Geometry: final body of the model. Coordinates: model frame, mm. Face numbers are marked on the shaded views. Round coordinates to 2 decimals unless told otherwise and drop trailing zeros. Loops run counter-clockwise (first coordinate to the right, second up) from the corner with the lowest first, then second, coordinate; pieces in that order, holes last. Notation, with made-up numbers: (1, -15.5) - (54, -15.5) arc R20 cw to (54, 15.5) - close; hole circle Ø11 at (-19, -31.75). An arc over 180 degrees is marked (long way). Answer as CSV lines item,"result".
from build123d import *

# Parameters (mm, degrees)
BOSS_EXTRUDE1_DEPTH = 2.5
SKETCH3_R           = 2.25
SKETCH3_R_2         = 2.1
SKETCH3_R_3         = 2.121320344
CUT_EXTRUDE1_DEPTH  = 3
SKETCH4_R           = 33.5
SKETCH4_R_2         = 2.25
CUT_EXTRUDE2_DEPTH  = 5
CUT_EXTRUDE3_DEPTH  = 1.5
CHAMFER1_SIZE       = 2
CUT_EXTRUDE4_DEPTH  = 3
SKETCH7_R           = 2.25
SKETCH7_R_2         = 1.25
BOSS_EXTRUDE2_DEPTH = 3
CHAMFER2_SIZE       = 2
SKETCH12_W          = 9
SKETCH12_H          = 42.1
CUT_EXTRUDE5_DEPTH  = 7
CHAMFER3_SIZE       = 0.4


with BuildPart() as part:
    # Sketch1 → Boss-Extrude1 (new body)
    with BuildSketch(Plane.XY):
        with BuildLine():
            Line((-15.633211847, 85.984955899), (119.366788153, 85.984955899))
            ThreePointArc((119.366788153, 85.984955899), (126.437855965, 83.05602371), (129.366788153, 75.984955899))
            Line((129.366788153, 75.984955899), (129.366788153, 10.984955899))
            ThreePointArc((129.366788153, 10.984955899), (126.437855965, 3.913888087), (119.366788153, 0.984955899))
            Line((119.366788153, 0.984955899), (-15.633211847, 0.984955899))
            ThreePointArc((-15.633211847, 0.984955899), (-22.704279659, 3.913888087), (-25.633211847, 10.984955899))
            Line((-25.633211847, 10.984955899), (-25.633211847, 75.984955899))
            ThreePointArc((-25.633211847, 75.984955899), (-22.704279659, 83.05602371), (-15.633211847, 85.984955899))
        make_face()
    extrude(amount=BOSS_EXTRUDE1_DEPTH)

    # Sketch3 → Cut-Extrude1 (cut)
    with BuildSketch(Plane.XY.offset(2.5)):
        with Locations((119.266788153, 11.084955899)):
            Circle(SKETCH3_R)
        with Locations((119.266788153, 75.984955899)):
            Circle(SKETCH3_R_2)
        with Locations((-15.533211847, 75.984955899)):
            Circle(SKETCH3_R_3)
        with Locations((-15.533211847, 11.084955899)):
            Circle(SKETCH3_R_2)
    extrude(amount=-CUT_EXTRUDE1_DEPTH, mode=Mode.SUBTRACT)

    # Sketch4 → Cut-Extrude2 (cut)
    with BuildSketch(Plane.XY.offset(2.5)):
        with Locations((58.842502754, 40.410046739)):
            Circle(SKETCH4_R)
        with Locations((28.842502754, 70.410046739)):
            Circle(SKETCH4_R_2)
        with Locations((88.842502754, 70.410046739)):
            Circle(SKETCH4_R_2)
        with Locations((88.842502754, 10.410046739)):
            Circle(SKETCH4_R_2)
        with Locations((28.842502754, 10.410046739)):
            Circle(SKETCH4_R_2)
    extrude(amount=-CUT_EXTRUDE2_DEPTH, mode=Mode.SUBTRACT)

    # Sketch5 → Cut-Extrude3 (cut)
    with BuildSketch(Plane(origin=(0, 0, 0), x_dir=(-1, 0, 0), z_dir=(0, 0, -1))):
        Polygon((-93.172629773, 10.410046739), (-91.007566263, 6.660046739), (-86.677439244, 6.660046739), (-84.512375735, 10.410046739), (-86.677439244, 14.160046739), (-91.007566263, 14.160046739), align=None)
        Polygon((-33.172629773, 10.410046739), (-31.007566263, 6.660046739), (-26.677439244, 6.660046739), (-24.512375735, 10.410046739), (-26.677439244, 14.160046739), (-31.007566263, 14.160046739), align=None)
        Polygon((-93.172629773, 70.410046739), (-91.007566263, 66.660046739), (-86.677439244, 66.660046739), (-84.512375735, 70.410046739), (-86.677439244, 74.160046739), (-91.007566263, 74.160046739), align=None)
        Polygon((-33.172629773, 70.410046739), (-31.007566263, 66.660046739), (-26.677439244, 66.660046739), (-24.512375735, 70.410046739), (-26.677439244, 74.160046739), (-31.007566263, 74.160046739), align=None)
    extrude(amount=-CUT_EXTRUDE3_DEPTH, mode=Mode.SUBTRACT)

    # Chamfer1
    chamfer1_edges = [part.edges().sort_by_distance(p)[0] for p in [
        (25.342502754, 40.410046739, 0),
    ]]
    chamfer(chamfer1_edges, length=CHAMFER1_SIZE)

    # Sketch6 → Cut-Extrude4 (cut)
    with BuildSketch(Plane.XY.offset(2.5)):
        with BuildLine():
            Line((20.342502754, 4.410046739), (20.342502754, 0.984955899))
            ThreePointArc((20.342502754, 0.984955899), (18.842502754, -0.515044101), (17.342502754, 0.984955899))
            Line((17.342502754, 0.984955899), (17.342502754, 4.410046739))
            ThreePointArc((17.342502754, 4.410046739), (18.842502754, 5.910046739), (20.342502754, 4.410046739))
        make_face()
    extrude(amount=-CUT_EXTRUDE4_DEPTH, mode=Mode.SUBTRACT)

    # Sketch7 → Boss-Extrude2 (add)
    # profile 1 of 2: a face of its own
    with BuildSketch(Plane(origin=(0, 0, 0), x_dir=(-1, 0, 0), z_dir=(0, 0, -1))):
        with Locations(Location((18.233971147, 25.069955899, 0), (0, 0, 180))):
            Circle(SKETCH7_R)
        with Locations((18.233971147, 25.069955899)):
            Circle(SKETCH7_R_2, mode=Mode.SUBTRACT)
    # profile 2 of 2: a face of its own
    with BuildSketch(Plane(origin=(0, 0, 0), x_dir=(-1, 0, 0), z_dir=(0, 0, -1))):
        with Locations(Location((1.723971147, 25.069955899, 0), (0, 0, 180))):
            Circle(SKETCH7_R)
        with Locations((1.723971147, 25.069955899)):
            Circle(SKETCH7_R_2, mode=Mode.SUBTRACT)
    extrude(amount=BOSS_EXTRUDE2_DEPTH)

    # Chamfer2
    chamfer2_edges = [part.edges().sort_by_distance(p)[0] for p in [
        (-20.483971147, 25.069955899, 0),
        (-3.973971147, 25.069955899, 0),
    ]]
    chamfer(chamfer2_edges, length=CHAMFER2_SIZE)

    # Sketch12 → Cut-Extrude5 (cut)
    with BuildSketch(Plane.XY.offset(2.5)):
        with Locations((109.912689541, 42.984621363)):
            Rectangle(SKETCH12_W, SKETCH12_H)
    extrude(amount=-CUT_EXTRUDE5_DEPTH, mode=Mode.SUBTRACT)

    # Chamfer3
    chamfer3_edges = [part.edges().sort_by_distance(p)[0] for p in [
        (105.412689541, 42.984621363, 2.5),
        (109.912689541, 21.934621363, 2.5),
        (114.412689541, 42.984621363, 2.5),
        (109.912689541, 64.034621363, 2.5),
        (25.342502754, 40.410046739, 2.5),
    ]]
    chamfer(chamfer3_edges, length=CHAMFER3_SIZE)


solid = part.part
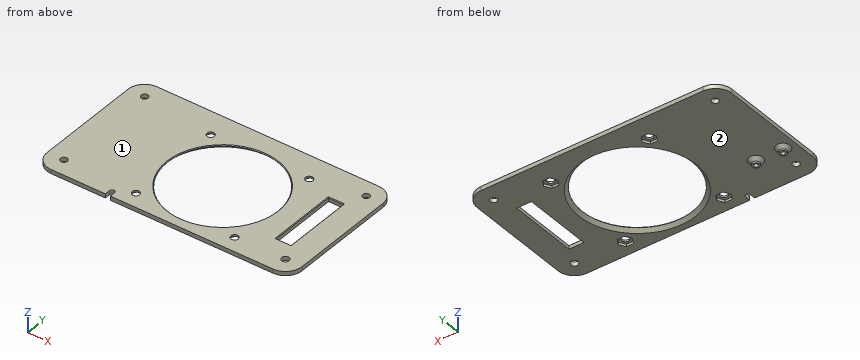
(1) Pin query (flat end, axial travel): P1, Ø5, axis at x = -15.53, y = 11.08, coming from the -Z side; P2, Ø2.5, axis at x = -15.53, y = 75.98, coming from the -Z side; P3, Ø2, axis at x = 30.5, y = 11, coming from the -Z side. Return the tip coordinate at first contact, or that it passes through.
Findings below:
P1,"z = 0"
P2,"through"
P3,"z = 1.5"
(2) Section B-B (x = 12). Output: boundary loops of the cut face in (y, z), and give its area (4 significant figures).
Findings below:
outline,"(0.98, 0) - (85.98, 0) - (85.98, 2.5) - (0.98, 2.5) - close"
area,"212.5 mm2"
(3) Section A-A (y = 45). Give the number of separate pieces and of enclosed holes in the cut face, and give its area (3 significant figures).
Findings below:
separate pieces,"3"
enclosed holes,"0"
area,"195 mm2"
(4) Material intervals for line 1 along Y through (x, z) = (106, 1.8); line 2 along X through (y, z) = (41, 0.3); line 3 along X through (y, z) = (36.5, 0.7), sorted ascending.
Findings below:
line 1,"0.98 to 21.93, 64.03 to 85.98"
line 2,"-25.63 to 23.65, 94.04 to 105.41, 114.41 to 129.37"
line 3,"-25.63 to 24.26, 93.42 to 105.41, 114.41 to 129.37"
(5) Draft query along Z for the marked faces 1 and 2. Return one class per face: pulls with the +Z half, pulls with the -Z half, needs draft (parallel to the pull), parting line crosses it, or undercut.
Findings below:
face 1,"pulls with the +Z half"
face 2,"pulls with the -Z half"
